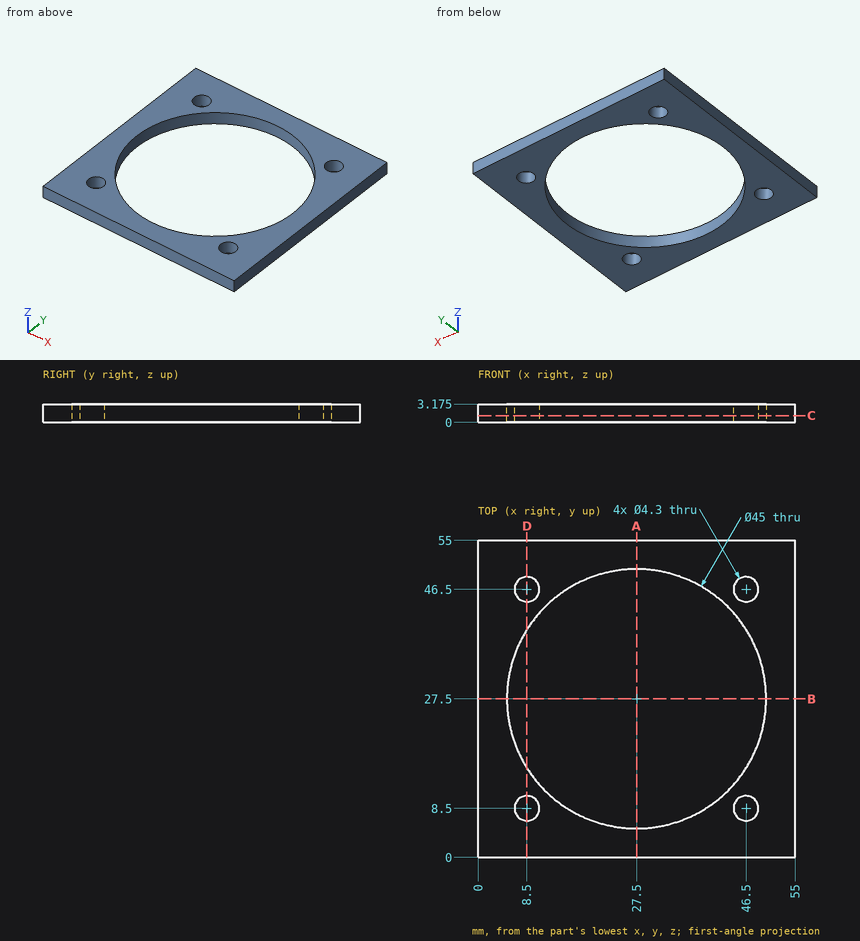
Verification items for this drawing (mm, ordinates from the low corner). Coordinates: 2 decimals unless noted, no trailing zeros. Write each loop counter-clockwise with the first axis right and the second up, starting at its lowest first coordinate (ties: lowest second). Pieces come first, ordered by that corner, then holes. Notation, with made-up numbers: M 44,47.25 L 73,47.25 A16 cw 73,66.25 Z; hole C 78,25.25 d5. An arc over 180 degrees is marked long. One line per item, written item: value. Start each with the question number.
(1) Depth check by flat-ended pin: pin 1 (5.5 mm diameter, centred on x = 46.5, y = 46.5, fed in from +Z) (3 decimals). Enter the tip coordinate at first touch or a pass-through.
(2) Scan lines: line 1 along X through (y, z) = (8.5, 0.75); line 2 along X through (y, z) = (31.5, 2.2). Record each from-to range of solid material in increasing order. Write a range as [from, to].
(3) Sectioned sample at D-D, the plane x = 8.5. Enter the section's corners in (y, z) (3 decimals).
(4) Sectioned sample at C-C, the plane z = 1.15. Enter the section's corners in (x, y), and give its area (3 significant figures).
(5) Sectioned sample at A-A, the plane x = 27.5. Enter the section's corners in (y, z) (3 decimals).
Filled sheet:
1. pin 1: z = 3.175
2. line 1: [0, 6.35], [10.65, 15.45], [39.55, 44.35], [48.65, 55]
2. line 2: [0, 5.36], [49.64, 55]
3. outline: M 0,0 L 6.35,0 L 6.35,3.175 L 0,3.175 Z; M 10.65,0 L 15.448,0 L 15.448,3.175 L 10.65,3.175 Z; M 39.552,0 L 44.35,0 L 44.35,3.175 L 39.552,3.175 Z; M 48.65,0 L 55,0 L 55,3.175 L 48.65,3.175 Z
4. outline: M 0,0 L 55,0 L 55,55 L 0,55 Z; hole C 27.5,27.5 d45; hole C 8.5,8.5 d4.3; hole C 8.5,46.5 d4.3; hole C 46.5,8.5 d4.3; hole C 46.5,46.5 d4.3
4. area: 1,380 mm²
5. outline: M 0,0 L 5,0 L 5,3.175 L 0,3.175 Z; M 50,0 L 55,0 L 55,3.175 L 50,3.175 Z
